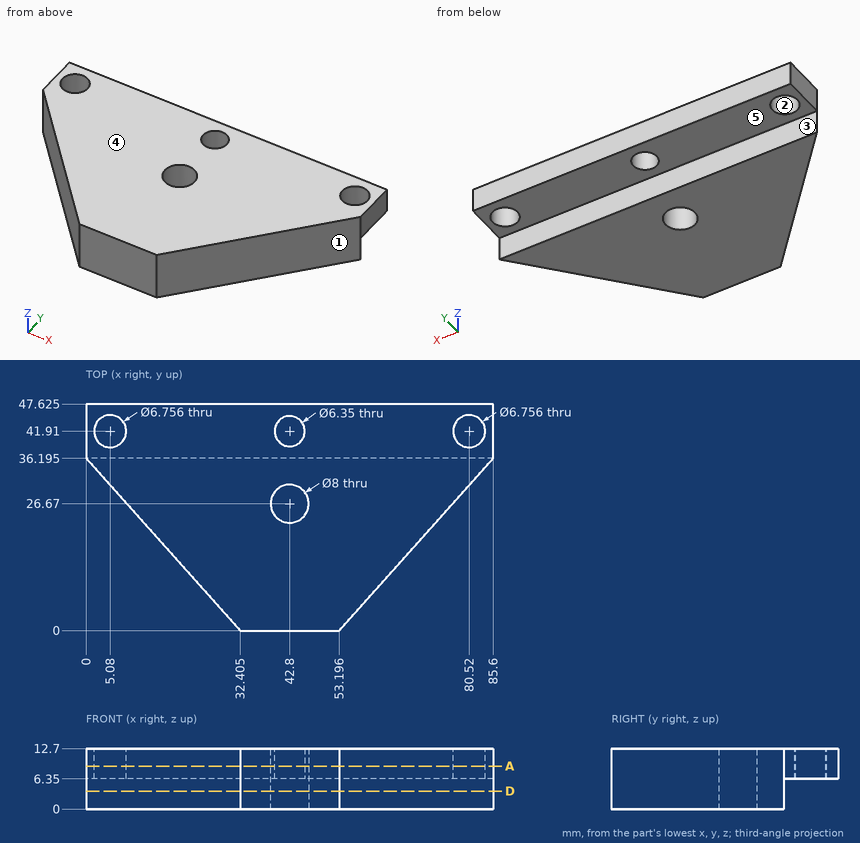
Can you work these out from the drawing? Everything is in mm from the part's minimum corner. A direction names the side the tool comes from. Give positions to 0.01 mm unless a question says otherwise; leave off trailing zeros. Loops run counter-clockwise (first coordinate to the right, second up) from the corner with the lowest first, then second, coordinate; pieces in that order, holes last. Notation, with made-up numbers: (81, 37) -> (92, 37) arc R17 ccw to (92, 45) -> close; hole circle Ø8 at (-7.5, -23). An arc over 180 degrees is marked (long way). Put each result on its own line as item: value.
(1) Please list where these lines run through material, in increasing order: probe 1 along Y at (x, z) = (5.08, 8.25) (1 decimal); probe 2 along Y at (x, z) = (5, 12.25) (1 decimal); probe 3 along X at (y, z) = (23, 4) (1 decimal). Write a range as [from, to].
Computed:
probe 1: [30.5, 38.5], [45.3, 47.6]
probe 2: [30.6, 38.5], [45.3, 47.6]
probe 3: [11.8, 41.2], [44.4, 73.8]
(2) For the marked faces 4 and 5, which set-ups out of +Z, -Z, +X, -X, +Y, -Y let a thin tool reach every point of the face, with its end or its side?
Computed:
face 4: +Z, +X, -X, +Y, -Y
face 5: -Z, +X, -X, +Y
(3) Imagine slicing it at D-D on z = 3.75. Write out the boundary of the cut face in (x, y) (1 decimal), plus the area to 4 significant figures.
Computed:
outline: (0, 36.2) -> (32.4, 0) -> (53.2, 0) -> (85.6, 36.2) -> close; hole circle Ø8 at (42.8, 26.7)
area: 1,875 mm^2
(4) I'm going to push flat-ended pins straight in: pin 1 Ø8 at (x, y) = (80.52, 41.91) entering from -Z; pin 2 Ø1.9 at (x, z) = (29, 3.5) entering from +Y (3 decimals); pin 3 Ø6 at (x, y) = (45.5, 41) entering from -Z; pin 4 Ø4 at (x, y) = (42.8, 41.91) entering from -Z. Where does each tip first touch, or does it pass through?
Computed:
pin 1: z = 6.35
pin 2: y = 36.195
pin 3: z = 6.35
pin 4: through
(5) Thinking about a two-plate mould opening in Y: for the marked faces 1, 2 and 3, which applies, pulls with the +Y half, pulls with the -Y half, needs draft (parallel to the pull), parting line crosses it, or undercut?
Computed:
face 1: pulls with the -Y half
face 2: undercut
face 3: pulls with the +Y half
(6) Imagine slicing it at A-A on z = 9. State how many separate pieces and enclosed holes the cut face has, plus the area to 3 significant figures.
Computed:
separate pieces: 1
enclosed holes: 4
area: 2,750 mm^2
